Design review of the part built by this model. Coordinates are the model's own, in mm. A direction names the side the tool comes from. Round coordinates to 2 decimals unless told otherwise and drop trailing zeros. Order: outer loops, then holes, each group sorted by start corner. A loop starts at its lowest first (then second) coordinate and runs counter-clockwise, first axis right, second up. Notation, with made-up numbers: M 10.5,72.25 L 39.5,72.25 A23 cw 39.5,94.25 Z; hole C -38,61 d1. An arc over 180 degrees is marked long. Use a Markdown table: item, result. Add a question column.
(1) Take a section at D-D (z = 3.5). Write out the cut boundary in (x, y).
(2) For pin 1 (4 mm diameter, centred on y = 7, z = 4.5, fed in from +X); pin 2 (1 mm diameter, centred on y = 4.5, z = -14, fed in from -X); pin 3 (0.8 mm diameter, centred on x = -3.5, y = 6, fed in from +Z); pin 4 (3 mm diameter, centred on x = -8.5, z = -11.5, fed in from -Y), all flat-tipped, find the tip position at first contact; note any pin that passes through.
(3) Take a section at C-C (y = 7.25). Write out the cut boundary in (x, z).
(4) To check wall thickness, follow probe 1 along Z at (x, y) = (-12.75, 4); probe 2 along Z at (x, y) = (-13.25, 7.25); probe 3 along Z at (x, y) = (-3.25, 5.75). State the ranges of each line that lie inside material, in increasing order. Write a range as from..to.
(5) Machinability: for faces 1 (the face through (-2.361, 5, -16)), 2 (the face through (-4, 5, -14.621)), 3 (the face through (-12.45, 4.63, -10.03)), 4 (the face through (-10, 4.634, 13.405)), which of the approach directions +Z, -Z, +X, -X, +Y, -Y give a long, thin tool a straight path to every point of the face, cutting with its end or side? Answer none if there is none.
(6) Take a section at A-A (x = -7.5). Write out the cut boundary in (y, z).
(7) The part is to be moulded in two halves that separate along Z. For faces 5 (the face through (-2.63, 4.77, -10.45)), 6 (the face through (-2.361, 5, -12)), 7 (the face through (-2.662, 4.766, -17.136)), say which applies: released by +Z, released by -Z, zero draft, split by the parting line, or undercut.
(8) Take a section at B-B (z = 12). Write out the cut boundary in (x, y), then the cut area to 3 significant figures.
```python
from build123d import *

# Parameters (mm, degrees)
ESTRUSIONE_ESTRUSIONE1_DEPTH = 9.4
RACCORDO1_R                  = 1


with BuildPart() as part:
    # Schizzo1 → Estrusione-Estrusione1 (new body)
    with BuildSketch(Plane(origin=(0, 0, 0), x_dir=(1, 0, 0), z_dir=(0, 1, 0))):
        with BuildLine():
            Line((-2.361490309, 17.420855221), (-14.691490309, 17.420855221))
            Line((-14.691490309, 17.420855221), (-14.691490309, 14.620855221))
            Line((-14.691490309, 14.620855221), (-12.011490309, 14.620855221))
            Line((-12.011490309, 14.620855221), (-12.011490309, 12.520855221))
            Line((-12.011490309, 12.520855221), (-14.691490309, 12.520855221))
            Line((-14.691490309, 12.520855221), (-14.691490309, 10.220855221))
            ThreePointArc((-14.691490309, 10.220855221), (-12.885979413, 10.061873727), (-11.076490309, 9.957499929))
            Line((-11.076490309, 9.957499929), (-11.076490309, 7.220855221))
            Line((-11.076490309, 7.220855221), (-17.319309854, -1.781905696))
            ThreePointArc((-17.319309854, -1.781905696), (-10.857687466, -18.322109867), (2.024570257, -6.100066099))
            Line((2.024570257, -6.100066099), (-2.842159863, -7.246773536))
            ThreePointArc((-2.842159863, -7.246773536), (-9.772569078, -13.461151023), (-13.402257337, -4.889428758))
            Line((-13.402257337, -4.889428758), (-5.976490309, 7.220855221))
            Line((-5.976490309, 7.220855221), (-5.976490309, 9.957499929))
            ThreePointArc((-5.976490309, 9.957499929), (-4.167001204, 10.061873727), (-2.361490309, 10.220855221))
            Line((-2.361490309, 10.220855221), (-2.361490309, 12.520855221))
            Line((-2.361490309, 12.520855221), (-5.041490309, 12.520855221))
            Line((-5.041490309, 12.520855221), (-5.041490309, 14.620855221))
            Line((-5.041490309, 14.620855221), (-2.361490309, 14.620855221))
            Line((-2.361490309, 14.620855221), (-2.361490309, 17.420855221))
        make_face()
    extrude(amount=ESTRUSIONE_ESTRUSIONE1_DEPTH)

    # Raccordo1
    raccordo1_edges = [part.edges().sort_by_distance(p)[0] for p in [
        (-2.842159863, 4.7, 7.246773536),
        (2.024570257, 4.7, 6.100066099),
        (-14.691490309, 4.7, -10.220855221),
        (-14.691490309, 4.7, -17.420855221),
        (-2.361490309, 4.7, -17.420855221),
        (-2.361490309, 4.7, -10.220855221),
    ]]
    fillet(raccordo1_edges, radius=RACCORDO1_R)


solid = part.part
```
Verdict:
| question | item | result |
|---|---|---|
| 1 | outline | M -18.29,0 L -12.55,0 L -12.55,9.4 L -18.29,9.4 Z |
| 2 | pin 1 | stops at x = 1.71 |
| 2 | pin 2 | stops at x = -12.01 |
| 2 | pin 3 | stops at z = 17.53 |
| 2 | pin 4 | stops at y = 0 |
| 3 | outline | M -17.32,1.78 L -11.08,-7.22 L -11.08,-9.96 A60 ccw -13.78,-10.13 A1 ccw -14.69,-11.13 L -14.69,-12.52 L -12.01,-12.52 L -12.01,-14.62 L -14.69,-14.62 L -14.69,-16.42 A1 ccw -13.69,-17.42 L -3.36,-17.42 A1 ccw -2.36,-16.42 L -2.36,-14.62 L -5.04,-14.62 L -5.04,-12.52 L -2.36,-12.52 L -2.36,-11.13 A1 ccw -3.27,-10.13 A60 ccw -5.98,-9.96 L -5.98,-7.22 L -13.4,4.89 A5.72 cw long -2.81,8.01 A1 ccw -2.04,7.06 L 0.93,6.36 A1 ccw 2.16,7.28 A10.7 ccw long Z |
| 4 | probe 1 | z = -17.42..-14.62, -12.52..-10.05, -4.81..3.83, 11.74..17.71 |
| 4 | probe 2 | z = -17.42..-14.62, -12.52..-10.09, -4.09..4.64, 11.1..17.48 |
| 4 | probe 3 | z = -17.41..-14.62, -12.52..-10.14, 10.09..17.19 |
| 5 | face 1 | -Z, +X, +Y, -Y |
| 5 | face 2 | +X, +Y, -Y |
| 5 | face 3 | -X, +Y, -Y |
| 5 | face 4 | +Y, -Y |
| 6 | outline | M 0,-17.42 L 9.4,-17.42 L 9.4,-4.74 L 0,-4.74 Z; M 0,13.51 L 9.4,13.51 L 9.4,18.53 L 0,18.53 Z |
| 7 | face 5 | undercut |
| 7 | face 6 | zero draft |
| 7 | face 7 | released by -Z |
| 8 | outline | M -18.4,0 L -12.49,0 L -12.49,9.4 L -18.4,9.4 Z; M -4.56,0 L 1.35,0 L 1.35,9.4 L -4.56,9.4 Z |
| 8 | area | 111 mm^2 |
